Design review of the part built by this model. Coordinates are the model's own, in mm. A direction names the side the tool comes from. Coordinates: 2 decimals unless noted, no trailing zeros. Loops run counter-clockwise (first coordinate to the right, second up) from the corner with the lowest first, then second, coordinate; pieces in that order, holes last. Notation, with made-up numbers: M -17,44.25 L 9,44.25 A23 cw 9,71.25 Z; hole C 41,22 d2. An arc over 180 degrees is marked long. One line per item, written item: value.
```python
from build123d import *

# Parameters (mm, degrees)
EXTRUDE1_DEPTH = 4.4
SKETCH3_R      = 1.1
EXTRUDE2_DEPTH = 15


with BuildPart() as part:
    # Sketch1 → Extrude1 (new body)
    with BuildSketch(Plane.XY):
        Polygon((3.5, -2.020725942), (3.5, 2.020725942), (0, 4.041451884), (-3.5, 2.020725942), (-3.5, -2.020725942), (0, -4.041451884), align=None)
    extrude(amount=EXTRUDE1_DEPTH)

    # Sketch2 → Revolve1 (revolve)
    with BuildSketch(Plane(origin=(0, 0, 0), x_dir=(0, 0, -1), z_dir=(1, 0, 0))):
        Polygon((-14.4, 0), (-14.4, 1.3), (-11.4, 1.3), (-11.4, 2), (-4.4, 2), (-4.4, 0), align=None)
    revolve(axis=Axis((0, 0, 4.4), (0, 0, 1)))

    # Sketch3 → Extrude2 (add)
    with BuildSketch(Plane(origin=(0, 0, 0), x_dir=(1, 0, 0), z_dir=(0, 1, 0))):
        with Locations(Location((0, -2.2, 0), (0, 0, 270))):
            Circle(SKETCH3_R)
    extrude(amount=-EXTRUDE2_DEPTH)


solid = part.part
```
(1) We need section A-A on z = 2.2. State the section outline as (x, y) points.
Reply:
outline: M -3.5,-2.02 L -1.1,-3.41 L -1.1,-15 L 1.1,-15 L 1.1,-3.41 L 3.5,-2.02 L 3.5,2.02 L 0,4.04 L -3.5,2.02 Z
(2) We need section C-C on y = -6.25. State the section outline as (x, z) points.
Reply:
outline: C 0,2.2 d2.2
(3) We need section D-D on z = 5.5. State the section outline as (x, y) points, then the cut area to 3 significant figures.
Reply:
outline: C 0,0 d4
area: 12.6 mm2
(4) Insertion check: pin 1 (4 mm diameter, centred on x = -2, y = -5.5, fed in from -Z); pin 2 (2 mm diameter, centred on x = 2, z = 2, fed in from -Y); pin 3 (4 mm diameter, centred on x = -3, z = 3.5, fed in from -Y); pin 4 (3 mm diameter, centred on x = 2, z = 8.5, fed in from +Y). Each pin has a flat end and moves straight along its axis. Give the tip position at first contact, or say it passes through.
Reply:
pin 1: stops at z = 1.1
pin 2: stops at y = -15
pin 3: stops at y = -3.46
pin 4: stops at y = 1.94
(5) We need section B-B on y = 0. State the section outline as (x, z) points.
Reply:
outline: M -3.5,0 L 3.5,0 L 3.5,4.4 L 2,4.4 L 2,11.4 L 1.3,11.4 L 1.3,14.4 L -1.3,14.4 L -1.3,11.4 L -2,11.4 L -2,4.4 L -3.5,4.4 Z
(6) Tool access review of faces 1 (the cylindrical face through (0.33, -9.11, 3.25)), 2 (the flat face through (0, 0, 14.4)), 3 (the cylindrical face through (-1.29, -0.17, 12.88)): name each direction out of +Z, -Z, +X, -X, +Y, -Y from which nothing blocks a thin tool from reaching the whole face with its end or side.
Reply:
face 1: -Y
face 2: +Z, +X, -X, +Y, -Y
face 3: +Z
(7) To check wall thickness, follow line 1 along Z through (x, y) = (0, -13); line 2 along Z through (x, y) = (3.25, 1); line 3 along X through (y, z) = (-3.5, 2.5). State the ranges of each line that lie inside material, in increasing order. Write a range as [from, to].
Reply:
line 1: z = [1.1, 3.3]
line 2: z = [0, 4.4]
line 3: x = [-1.06, 1.06]
